```python
from build123d import *

# Parameters (mm, degrees)
SKETCH1_R                 = 3.4
F_40_X_40L_X_R4_5_1_DEPTH = 429


with BuildPart() as part:
    # Sketch1 → 铝型材 40 X 40L X R4.5(1) (new body)
    with BuildSketch(Plane(origin=(-12.168141593, 0, 0), x_dir=(0, 0, -1), z_dir=(1, 0, 0))):
        with BuildLine():
            Line((-5.1, 20), (-5.1, 19.5))
            Line((-5.1, 19.5), (-4.1, 19.5))
            Line((-4.1, 19.5), (-4.1, 17))
            Line((-4.1, 17), (-6.1, 17))
            Line((-6.1, 17), (-6.1, 18.5))
            Line((-6.1, 18.5), (-10.3, 18.5))
            Line((-10.3, 18.5), (-10.3, 11.3))
            Line((-10.3, 11.3), (-5, 6))
            Line((-5, 6), (5, 6))
            Line((5, 6), (10.3, 11.3))
            Line((10.3, 11.3), (10.3, 18.5))
            Line((10.3, 18.5), (6.1, 18.5))
            Line((6.1, 18.5), (6.1, 17))
            Line((6.1, 17), (4.1, 17))
            Line((4.1, 17), (4.1, 19.5))
            Line((4.1, 19.5), (5.1, 19.5))
            Line((5.1, 19.5), (5.1, 20))
            Line((5.1, 20), (15.5, 20))
            ThreePointArc((15.5, 20), (18.681980515, 18.681980515), (20, 15.5))
            Line((20, 15.5), (20, 5.1))
            Line((20, 5.1), (19.5, 5.1))
            Line((19.5, 5.1), (19.5, 4.1))
            Line((19.5, 4.1), (17, 4.1))
            Line((17, 4.1), (17, 6.1))
            Line((17, 6.1), (18.5, 6.1))
            Line((18.5, 6.1), (18.5, 10.3))
            Line((18.5, 10.3), (11.3, 10.3))
            Line((11.3, 10.3), (6, 5))
            Line((6, 5), (6, -5))
            Line((6, -5), (11.3, -10.3))
            Line((11.3, -10.3), (18.5, -10.3))
            Line((18.5, -10.3), (18.5, -6.1))
            Line((18.5, -6.1), (17, -6.1))
            Line((17, -6.1), (17, -4.1))
            Line((17, -4.1), (19.5, -4.1))
            Line((19.5, -4.1), (19.5, -5.1))
            Line((19.5, -5.1), (20, -5.1))
            Line((20, -5.1), (20, -15.5))
            ThreePointArc((20, -15.5), (18.681980515, -18.681980515), (15.5, -20))
            Line((15.5, -20), (5.1, -20))
            Line((5.1, -20), (5.1, -19.5))
            Line((5.1, -19.5), (4.1, -19.5))
            Line((4.1, -19.5), (4.1, -17))
            Line((4.1, -17), (6.1, -17))
            Line((6.1, -17), (6.1, -18.5))
            Line((6.1, -18.5), (10.3, -18.5))
            Line((10.3, -18.5), (10.3, -11.3))
            Line((10.3, -11.3), (5, -6))
            Line((5, -6), (-5, -6))
            Line((-5, -6), (-10.3, -11.3))
            Line((-10.3, -11.3), (-10.3, -18.5))
            Line((-10.3, -18.5), (-6.1, -18.5))
            Line((-6.1, -18.5), (-6.1, -17))
            Line((-6.1, -17), (-4.1, -17))
            Line((-4.1, -17), (-4.1, -19.5))
            Line((-4.1, -19.5), (-5.1, -19.5))
            Line((-5.1, -19.5), (-5.1, -20))
            Line((-5.1, -20), (-15.5, -20))
            ThreePointArc((-15.5, -20), (-18.681980515, -18.681980515), (-20, -15.5))
            Line((-20, -15.5), (-20, -5.1))
            Line((-20, -5.1), (-19.5, -5.1))
            Line((-19.5, -5.1), (-19.5, -4.1))
            Line((-19.5, -4.1), (-17, -4.1))
            Line((-17, -4.1), (-17, -6.1))
            Line((-17, -6.1), (-18.5, -6.1))
            Line((-18.5, -6.1), (-18.5, -10.3))
            Line((-18.5, -10.3), (-11.3, -10.3))
            Line((-11.3, -10.3), (-6, -5))
            Line((-6, -5), (-6, 5))
            Line((-6, 5), (-11.3, 10.3))
            Line((-11.3, 10.3), (-18.5, 10.3))
            Line((-18.5, 10.3), (-18.5, 6.1))
            Line((-18.5, 6.1), (-17, 6.1))
            Line((-17, 6.1), (-17, 4.1))
            Line((-17, 4.1), (-19.5, 4.1))
            Line((-19.5, 4.1), (-19.5, 5.1))
            Line((-19.5, 5.1), (-20, 5.1))
            Line((-20, 5.1), (-20, 15.5))
            ThreePointArc((-20, 15.5), (-18.681980515, 18.681980515), (-15.5, 20))
            Line((-15.5, 20), (-5.1, 20))
        make_face()
        Circle(SKETCH1_R, mode=Mode.SUBTRACT)
        with BuildLine():
            Line((11.8, 17.5), (15, 17.5))
            ThreePointArc((15, 17.5), (16.767766953, 16.767766953), (17.5, 15))
            Line((17.5, 15), (17.5, 11.8))
            Line((17.5, 11.8), (11.8, 11.8))
            Line((11.8, 11.8), (11.8, 17.5))
        make_face(mode=Mode.SUBTRACT)
        with BuildLine():
            Line((-15, 17.5), (-11.8, 17.5))
            Line((-11.8, 17.5), (-11.8, 11.8))
            Line((-11.8, 11.8), (-17.5, 11.8))
            Line((-17.5, 11.8), (-17.5, 15))
            ThreePointArc((-17.5, 15), (-16.767766953, 16.767766953), (-15, 17.5))
        make_face(mode=Mode.SUBTRACT)
        with BuildLine():
            Line((-17.5, -11.8), (-11.8, -11.8))
            Line((-11.8, -11.8), (-11.8, -17.5))
            Line((-11.8, -17.5), (-15, -17.5))
            ThreePointArc((-15, -17.5), (-16.767766953, -16.767766953), (-17.5, -15))
            Line((-17.5, -15), (-17.5, -11.8))
        make_face(mode=Mode.SUBTRACT)
        with BuildLine():
            Line((11.8, -11.8), (17.5, -11.8))
            Line((17.5, -11.8), (17.5, -15))
            ThreePointArc((17.5, -15), (16.767766953, -16.767766953), (15, -17.5))
            Line((15, -17.5), (11.8, -17.5))
            Line((11.8, -17.5), (11.8, -11.8))
        make_face(mode=Mode.SUBTRACT)
    extrude(amount=F_40_X_40L_X_R4_5_1_DEPTH)


solid = part.part
```
CAD build for the part. Positions are in the model's coordinates, mm. A direction names the side the tool comes from. Round coordinates to 2 decimals unless told otherwise and drop trailing zeros. Return JSON: item names as keys, results as strings. Group by question number.
Q1. Drill centre lines: line 1 along Z through (x, y) = (40, -13.5); line 2 along Z through (x, y) = (162, 5). Where is each one in solid material? Low to high. Write a range as [from, to].
Q2. Band-saw the part on A-A on x = 180.5. Give the number of separate pieces and of enclosed holes in the cut face, plus the area to 3 significant figures.
Q3. Flat gauge pins, fed straight in: pin 1 Ø3 at (x, y) = (151.5, 18) entering from +Z; pin 2 Ø1 at (x, y) = (336, 1.5) entering from -Z; pin 3 Ø2 at (y, z) = (13, -15.5) entering from +X; pin 4 Ø1.6 at (x, y) = (169, -18) entering from +Z. Where does each tip first touch, or does it go through?
Q4. Two-plate mould, pull along Z, no slides. Class faces 1 (the face through (199, -10, 20)), 2 (the face through (199, 20, 10)), 3 (the face through (199, 6, 0)): +Z half, -Z half, draft (parallel to the pull), parting line (faces both ways), or undercut.
Q5. Tool access for faces 4 (the face through (199, 0, 6)), 5 (the face through (199, -20, 10)): list every direction of +Z, -Z, +X, -X, +Y, -Y with a clear straight run to the whole face (end or side of a thin tool).
Solutions:
{
 "1": {"line 1": "z = [-20, -17.5], [-11.8, -10.3], [10.3, 11.8], [17.5, 20]", "line 2": "z = [-19.5, -17], [-6, 6], [17, 19.5]"},
 "2": {"separate pieces": "1", "enclosed holes": "5", "area": "475 mm^2"},
 "3": {"pin 1": "stops at z = 19.89", "pin 2": "stops at z = -6", "pin 3": "passes through", "pin 4": "stops at z = 19.67"},
 "4": {"face 1": "+Z half", "face 2": "draft", "face 3": "undercut"},
 "5": {"face 4": "+X, -X", "face 5": "+Z, -Z, +X, -X, -Y"}
}
